from build123d import *

# Parameters (mm, degrees)
SKETCH1_W               = 25.4
SKETCH1_H               = 25.4
EXTRUDE1_DEPTH          = 76.2
SKETCH2_W               = 19.05
SKETCH2_H               = 19.05
EXTRUDE2_DEPTH          = 154.454683865
F_3_8_CLEARANCE_HOLE1_D = 10.0838
F_3_8_CLEARANCE_HOLE2_D = 10.0838


with BuildPart() as part:
    # Sketch1 → Extrude1 (new, symmetric)
    with BuildSketch(Plane.XY):
        Rectangle(SKETCH1_W, SKETCH1_H)
    extrude(amount=EXTRUDE1_DEPTH, both=True)

    # Sketch2 → Extrude2 (cut, through all)
    with BuildSketch(Plane.XY.offset(76.2)):
        Rectangle(SKETCH2_W, SKETCH2_H)
    extrude(amount=-EXTRUDE2_DEPTH, mode=Mode.SUBTRACT)

    # 3/8 Clearance Hole1 (through all)
    with Locations(Plane(origin=(12.7, 0, 0), x_dir=(0, 0, -1), z_dir=(1, 0, 0))):
        with Locations((-63.5, 0)):
            f_3_8_clearance_hole1 = Hole(F_3_8_CLEARANCE_HOLE1_D / 2)

    # 3/8 Clearance Hole2 (through all)
    with Locations(Plane(origin=(0, 12.7, 0), x_dir=(-1, 0, 0), z_dir=(0, 1, 0))):
        with Locations((0, 50.8)):
            f_3_8_clearance_hole2 = Hole(F_3_8_CLEARANCE_HOLE2_D / 2)

    # Mirror1: 3/8 Clearance Hole1, 3/8 Clearance Hole2 across plane
    add(f_3_8_clearance_hole1.mirror(Plane.XY), mode=Mode.SUBTRACT)
    add(f_3_8_clearance_hole2.mirror(Plane.XY), mode=Mode.SUBTRACT)


solid = part.part
Model file for the job. Use its own axes, mm. A direction names the side the tool comes from. Give positions to 0.01 mm unless a question says otherwise; leave off trailing zeros. Order: outer loops, then holes, each group sorted by start corner. A loop starts at its lowest first (then second) coordinate and runs counter-clockwise, first axis right, second up. Notation, with made-up numbers: (-35, -19) - (-1, -19) arc R35 cw to (-1, 18) - close; hole circle Ø8 at (63, -38.5). An arc over 180 degrees is marked (long way). One line per item, written item: value.
Item 1: Slice it at D-D (z = -37). List the corners of the cut face in (x, y) (3 decimals).
Response values:
outline: (-12.7, -12.7) - (12.7, -12.7) - (12.7, 12.7) - (-12.7, 12.7) - close; hole (-9.525, -9.525) - (9.525, -9.525) - (9.525, 9.525) - (-9.525, 9.525) - close
Item 2: Tool access for faces 1 (the flat face through (0, -9.525, 1)), 2 (the flat face through (0, 12.7, 1)): list every direction of +Z, -Z, +X, -X, +Y, -Y with a clear straight run to the whole face (end or side of a thin tool).
Response values:
face 1: +Z, -Z
face 2: +Z, -Z, +X, -X, +Y
Item 3: Slice it at B-B (x = 0). List the corners of the cut face in (y, z) (3 decimals).
Response values:
outline: (-12.7, -76.2) - (-9.525, -76.2) - (-9.525, -55.842) - (-12.7, -55.842) - close; (-12.7, -45.758) - (-9.525, -45.758) - (-9.525, 45.758) - (-12.7, 45.758) - close; (-12.7, 55.842) - (-9.525, 55.842) - (-9.525, 76.2) - (-12.7, 76.2) - close; (9.525, -76.2) - (12.7, -76.2) - (12.7, -55.842) - (9.525, -55.842) - close; (9.525, -45.758) - (12.7, -45.758) - (12.7, 45.758) - (9.525, 45.758) - close; (9.525, 55.842) - (12.7, 55.842) - (12.7, 76.2) - (9.525, 76.2) - close
Item 4: Slice it at C-C (y = 0). List the corners of the cut face in (x, z) (3 decimals), then the cut area to 3 significant figures.
Response values:
outline: (-12.7, -76.2) - (-9.525, -76.2) - (-9.525, -68.542) - (-12.7, -68.542) - close; (-12.7, -58.458) - (-9.525, -58.458) - (-9.525, 58.458) - (-12.7, 58.458) - close; (-12.7, 68.542) - (-9.525, 68.542) - (-9.525, 76.2) - (-12.7, 76.2) - close; (9.525, -76.2) - (12.7, -76.2) - (12.7, -68.542) - (9.525, -68.542) - close; (9.525, -58.458) - (12.7, -58.458) - (12.7, 58.458) - (9.525, 58.458) - close; (9.525, 68.542) - (12.7, 68.542) - (12.7, 76.2) - (9.525, 76.2) - close
area: 840 mm2
Item 5: Slice it at A-A (z = 63.5). List the corners of the cut face in (x, y) (3 decimals).
Response values:
outline: (-12.7, -12.7) - (12.7, -12.7) - (12.7, -5.042) - (9.525, -5.042) - (9.525, -9.525) - (-9.525, -9.525) - (-9.525, -5.042) - (-12.7, -5.042) - close; (-12.7, 5.042) - (-9.525, 5.042) - (-9.525, 9.525) - (9.525, 9.525) - (9.525, 5.042) - (12.7, 5.042) - (12.7, 12.7) - (-12.7, 12.7) - close
Item 6: Wall check: line 1 (X direction, y = 6.5, z = -56) (3 decimals); line 2 (Z direction, x = 0, y = 10.4). Give the ranges that are in metal, low to high.
Response values:
line 1: -12.7 to -9.525, 9.525 to 12.7
line 2: -76.2 to -55.84, -45.76 to 45.76, 55.84 to 76.2
Item 7: Two-plate mould, pull along X, no slides. Class faces 3 (the flat face through (12.7, 0, 1)), 4 (the flat face through (0, -12.7, 1)), 5 (the cylindrical face through (2.71, 11.09, -55.05)): released by +X, released by -X, zero draft, split by the parting line, or undercut.
Response values:
face 3: released by +X
face 4: zero draft
face 5: undercut
